```python
from build123d import *

# Parameters (mm, degrees)
SKETCH1_W           = 900
SKETCH1_H           = 800
SKETCH1_W_2         = 5
SKETCH1_H_2         = 200
BOSS_EXTRUDE1_DEPTH = 10
SKETCH2_R           = 62.5
CUT_EXTRUDE4_DEPTH  = 196
SKETCH3_R           = 2
SKETCH3_W           = 36.55
SKETCH3_H           = 6
SKETCH3_W_2         = 240
SKETCH3_H_2         = 5
CUT_EXTRUDE5_DEPTH  = 11


with BuildPart() as part:
    # Sketch1 → Boss-Extrude1 (new body)
    with BuildSketch(Plane(origin=(0, 0, 0), x_dir=(1, 0, 0), z_dir=(0, 1, 0))):
        with Locations((50, -100)):
            Rectangle(SKETCH1_W, SKETCH1_H)
        with Locations((397.5, 180)):
            Rectangle(SKETCH1_W_2, SKETCH1_H_2, mode=Mode.SUBTRACT)
        with Locations((-297.5, 180)):
            Rectangle(SKETCH1_W_2, SKETCH1_H_2, mode=Mode.SUBTRACT)
        with Locations((-297.5, -380)):
            Rectangle(SKETCH1_W_2, SKETCH1_H_2, mode=Mode.SUBTRACT)
        with Locations((397.5, -380)):
            Rectangle(SKETCH1_W_2, SKETCH1_H_2, mode=Mode.SUBTRACT)
    extrude(amount=BOSS_EXTRUDE1_DEPTH)

    # Sketch2 → Cut-Extrude4 (cut)
    with BuildSketch(Plane(origin=(0, 0, 0), x_dir=(1, 0, 0), z_dir=(0, 1, 0))):
        with Locations((-300, -100)):
            Circle(SKETCH2_R)
    extrude(amount=CUT_EXTRUDE4_DEPTH, mode=Mode.SUBTRACT)

    # Sketch3 → Cut-Extrude5 (cut, through all)
    with BuildSketch(Plane(origin=(0, 0, 0), x_dir=(1, 0, 0), z_dir=(0, 1, 0))):
        with Locations((-296.5, -30)):
            Circle(SKETCH3_R)
        with Locations((-303.5, -30)):
            Circle(SKETCH3_R)
        with Locations((-303.5, -170)):
            Circle(SKETCH3_R)
        with Locations((-296.5, -170)):
            Circle(SKETCH3_R)
        with Locations((147.13212951, -115.75)):
            Rectangle(SKETCH3_W, SKETCH3_H)
        with Locations((147.13212951, -84.25)):
            Rectangle(SKETCH3_W, SKETCH3_H)
        with Locations((-80, -168.5)):
            Rectangle(SKETCH3_W_2, SKETCH3_H_2)
        with Locations((-80, -31.5)):
            Rectangle(SKETCH3_W_2, SKETCH3_H_2)
    extrude(amount=CUT_EXTRUDE5_DEPTH, mode=Mode.SUBTRACT)


solid = part.part
```
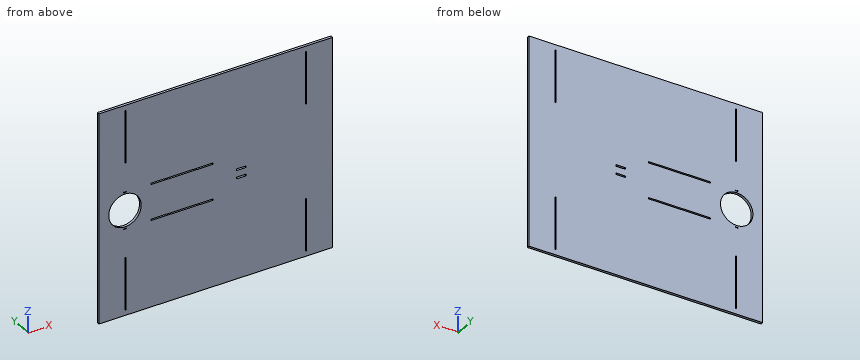
Build history of the part. All positions in model axes, mm. Round coordinates to 2 decimals unless told otherwise and drop trailing zeros. Order: outer loops, then holes, each group sorted by start corner. A loop starts at its lowest first (then second) coordinate and runs counter-clockwise, first axis right, second up. Notation, with made-up numbers: (57, -39.5) -> (97, -39.5) arc R24 cw to (97, -24.5) -> close; hole circle Ø5 at (2, -15). An arc over 180 degrees is marked (long way). Answer in a Markdown table with one row per item.
1) Band-saw the part on B-B on y = 4.5. Give the number of separate pieces and of enclosed holes in the cut face, and give its area (3 significant figures).
Values:
| item | result |
|---|---|
| separate pieces | 1 |
| enclosed holes | 13 |
| area | 701,000 mm2 |
2) Wall check: L1, parallel to X at y = 6.25, z = 410; L2, parallel to Z at x = -33, y = 0.75; L3, parallel to X at y = 2.5, z = 170. Give the ranges that are in metal, low to high.
Values:
| item | result |
|---|---|
| L1 | -400 to -300, -295 to 395, 400 to 500 |
| L2 | -300 to 29, 34 to 166, 171 to 500 |
| L3 | -400 to -305.5, -301.5 to -298.5, -294.5 to -200, 40 to 500 |
3) Band-saw the part on A-A on z = 100. Give the cut face in (x, y), and give its area (3 significant figures).
Values:
| item | result |
|---|---|
| outline | (-400, 0) -> (-362.5, 0) -> (-362.5, 10) -> (-400, 10) -> close; (-237.5, 0) -> (500, 0) -> (500, 10) -> (-237.5, 10) -> close |
| area | 7,750 mm2 |
